from build123d import *

# Parameters (mm, degrees)
F0_R     = 2.5
F1_DEPTH = 2
F0_R_2   = 1.5
F2_DEPTH = 10
F3_DEPTH = 2
F0_R_3   = 2
F4_DEPTH = 2
F5_DEPTH = 2


with BuildPart() as f1:
    # F0 (on Front) → F1 (new body)
    with BuildSketch(Plane.XZ):
        with BuildLine():
            ThreePointArc((9.7653447127, -2.1536115346), (8.9493655339, 0), (9.7653447127, 2.1536115346))
            ThreePointArc((9.7653447127, 2.1536115346), (-0.0002939612, 9.9999999957), (-9.7654713115, 2.1530374044))
            ThreePointArc((-9.7654713115, 2.1530374044), (-9.1606975934, 1.1511476366), (-8.95, 0))
            ThreePointArc((-8.95, 0), (-9.1606975934, -1.1511476366), (-9.7654713115, -2.1530374044))
            ThreePointArc((-9.7654713115, -2.1530374044), (-0.0002939612, -9.9999999957), (9.7653447127, -2.1536115346))
        make_face()
        with Locations((-4.5, 0)):
            Circle(F0_R, mode=Mode.SUBTRACT)
        with Locations((4.5, 0)):
            Circle(F0_R, mode=Mode.SUBTRACT)
    extrude(amount=F1_DEPTH)

    # F0 (on Front) → F2 (join)
    with BuildSketch(Plane.XZ):
        with Locations((-4.5, 0)):
            Circle(F0_R)
        with Locations((-4.5, 0)):
            Circle(F0_R_2, mode=Mode.SUBTRACT)
        with Locations((4.5, 0)):
            Circle(F0_R)
        with Locations((4.5, 0)):
            Circle(F0_R_2, mode=Mode.SUBTRACT)
    extrude(amount=F2_DEPTH)

    # F0 (on Front) → F3 (join)
    with BuildSketch(Plane.XZ):
        with BuildLine():
            ThreePointArc((9.7653447127, -2.1536115346), (8.9493655339, 0), (9.7653447127, 2.1536115346))
            ThreePointArc((9.7653447127, 2.1536115346), (-0.0002939612, 9.9999999957), (-9.7654713115, 2.1530374044))
            ThreePointArc((-9.7654713115, 2.1530374044), (-9.1606975934, 1.1511476366), (-8.95, 0))
            ThreePointArc((-8.95, 0), (-9.1606975934, -1.1511476366), (-9.7654713115, -2.1530374044))
            ThreePointArc((-9.7654713115, -2.1530374044), (-0.0002939612, -9.9999999957), (9.7653447127, -2.1536115346))
        make_face()
        with Locations((-4.5, 0)):
            Circle(F0_R, mode=Mode.SUBTRACT)
        with Locations((4.5, 0)):
            Circle(F0_R, mode=Mode.SUBTRACT)
    extrude(amount=F3_DEPTH)

    # F0 (on Front) → F4 (join)
    with BuildSketch(Plane.XZ):
        with BuildLine():
            ThreePointArc((9.7653447127, 2.1536115346), (9.9411630891, 1.0831788571), (10, 0))
            ThreePointArc((10, 0), (9.9411630891, -1.0831788571), (9.7653447127, -2.1536115346))
            ThreePointArc((9.7653447127, -2.1536115346), (13.3508715762, -3.0391666349), (15.4493655339, 0))
            ThreePointArc((15.4493655339, 0), (13.3508715762, 3.0391666349), (9.7653447127, 2.1536115346))
        make_face()
        with Locations((12.1999992313, 0.0043308363)):
            Circle(F0_R_3, mode=Mode.SUBTRACT)
        with BuildLine():
            ThreePointArc((-9.7654713115, -2.1530374044), (-10, 0), (-9.7654713115, 2.1530374044))
            ThreePointArc((-9.7654713115, 2.1530374044), (-15.45, 0), (-9.7654713115, -2.1530374044))
        make_face()
        with Locations((-12.2, 0)):
            Circle(F0_R_3, mode=Mode.SUBTRACT)
    extrude(amount=F4_DEPTH)

    # F0 (on Front) → F5 (join)
    with BuildSketch(Plane.XZ):
        with BuildLine():
            ThreePointArc((9.7653447127, -2.1536115346), (9.9411630891, -1.0831788571), (10, 0))
            ThreePointArc((10, 0), (9.9411630891, 1.0831788571), (9.7653447127, 2.1536115346))
            ThreePointArc((9.7653447127, 2.1536115346), (8.9493655339, 0), (9.7653447127, -2.1536115346))
        make_face()
        with BuildLine():
            ThreePointArc((-8.95, 0), (-9.1606975934, 1.1511476366), (-9.7654713115, 2.1530374044))
            ThreePointArc((-9.7654713115, 2.1530374044), (-10, 0), (-9.7654713115, -2.1530374044))
            ThreePointArc((-9.7654713115, -2.1530374044), (-9.1606975934, -1.1511476366), (-8.95, 0))
        make_face()
    extrude(amount=F5_DEPTH)


solid = f1.part
CAD build for the part. Positions are in the model's coordinates, mm. A direction names the side the tool comes from. Round coordinates to 2 decimals unless told otherwise and drop trailing zeros. Order: outer loops, then holes, each group sorted by start corner. A loop starts at its lowest first (then second) coordinate and runs counter-clockwise, first axis right, second up. Notation, with made-up numbers: M -37.5,39 L -31.5,39 A15 cw -31.5,64 Z; hole C 21,-36.75 d7. An arc over 180 degrees is marked long. Use one line per item in the form item = value.
Q1. Saw through at B-B on y = -4.25. Give the cut face in (x, z), then the cut area to 3 significant figures.
Recorded:
outline = C -4.5,0 d5; C 4.5,0 d5; hole C -4.5,0 d3; hole C 4.5,0 d3
area = 25.1 mm^2
Q2. Two-plate mould, pull along Z, no slides. Class faces 3 (the flat face through (0, -2, 0)), 4 (the cylindrical face through (-5.7, -4.9, -0.9)), 5 (the cylindrical face through (6.885, -5.944, 0.751)): +Z half, -Z half, draft (parallel to the pull), parting line (faces both ways), or undercut.
Recorded:
face_3 = draft
face_4 = undercut
face_5 = parting line
Q3. Which spindle directions (+Z, -Z, +X, -X, +Y, -Y) get a long thin tool onto all of the face, cutting with end or side? Do faces 1 (the cylindrical face through (-10.292, -0.986, 0.601)), 2 (the cylindrical face through (-2.115, -5.944, 0.751)). Say none if no direction does.
Recorded:
face_1 = +Y, -Y
face_2 = -Y
Q4. Saw through at D-D on x = 13. Give the cut face in (y, z), then the cut area to 3 significant figures.
Recorded:
outline = M -2,-3.15 L 0,-3.15 L 0,-1.83 L -2,-1.83 Z; M -2,1.84 L 0,1.84 L 0,3.15 L -2,3.15 Z
area = 5.27 mm^2
Q5. Saw through at C-C on y = -1. Give the cut face in (x, z).
Recorded:
outline = M -9.77,-2.15 A10 ccw 9.77,-2.15 A3.25 ccw long 9.77,2.15 A10 ccw -9.77,2.15 A3.25 ccw long Z; hole C -12.2,0 d4; hole C -4.5,0 d3; hole C 4.5,0 d3; hole C 12.2,0 d4
Q6. Saw through at A-A on x = -12.2. Give the cut face in (y, z), then the cut area to 3 significant figures.
Recorded:
outline = M -2,-3.25 L 0,-3.25 L 0,-2 L -2,-2 Z; M -2,2 L 0,2 L 0,3.25 L -2,3.25 Z
area = 5.00 mm^2
Q7. Probe L1, parallel to X at y = -7.75, z = -0.5; L2, parallel to Z at x = 4.5, y = -2.25; L3, parallel to Z at x = 12.2, y = -1.4. List the from-to ranges inside material, lowest first.
Recorded:
L1 = -6.95 to -5.91, -3.09 to -2.05, 2.05 to 3.09, 5.91 to 6.95
L2 = -2.5 to -1.5, 1.5 to 2.5
L3 = -3.25 to -2, 2 to 3.25
Q8. Flat gauge pins, fed straight in: P1, Ø1.5, axis at x = -8.5, z = 1, coming from the -Y side; P2, Ø6.5, axis at x = 12.2, z = 0, coming from the +Y side; P3, Ø5, axis at y = -7, z = -6, coming from the +X side; P4, Ø6, axis at y = -2, z = -7, coming from the +X side. Where does each tip first touch, or does it go through?
Recorded:
P1 = -2
P2 = 0
P3 = through
P4 = 9.17
